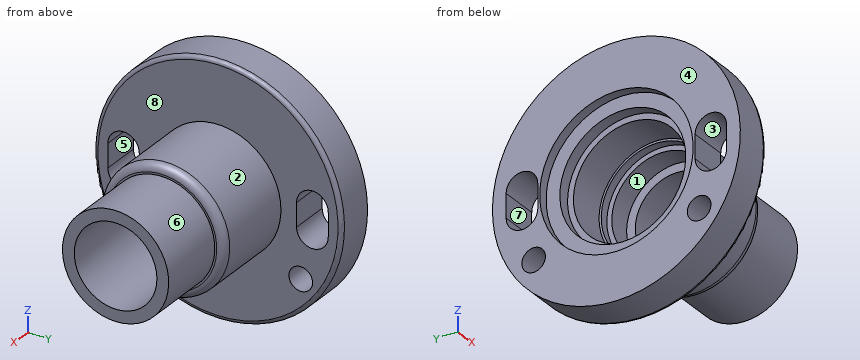
```python
from build123d import *

# Parameters (mm, degrees)
SKETCH1_R           = 31.5
BOSS_EXTRUDE1_DEPTH = 10
SKETCH2_R           = 16
BOSS_EXTRUDE2_DEPTH = 22
SKETCH3_R           = 13.5
BOSS_EXTRUDE3_DEPTH = 18
FILLET1_R           = 1
FILLET6_R           = 2
SKETCH4_R           = 10.5
CUT_EXTRUDE1_DEPTH  = 150
SKETCH5_R           = 12.7
CUT_EXTRUDE2_DEPTH  = 23.5
SKETCH6_R           = 13.95
CUT_EXTRUDE3_DEPTH  = 17.7
SKETCH7_R           = 14.5
CUT_EXTRUDE4_DEPTH  = 15.5
SKETCH8_R           = 16
CUT_EXTRUDE5_DEPTH  = 5.5
SKETCH9_R           = 19.5
CUT_EXTRUDE6_DEPTH  = 2.5
SKETCH10_R          = 3
CUT_EXTRUDE11_DEPTH = 20
SKETCH11_R          = 3
CUT_EXTRUDE12_DEPTH = 20
CUT_EXTRUDE16_DEPTH = 20
CUT_EXTRUDE17_DEPTH = 20


with BuildPart() as part:
    # Sketch1 → Boss-Extrude1 (new body)
    with BuildSketch(Plane(origin=(0, 0, 0), x_dir=(0, 0, -1), z_dir=(1, 0, 0))):
        Circle(SKETCH1_R)
    extrude(amount=BOSS_EXTRUDE1_DEPTH)

    # Sketch2 → Boss-Extrude2 (add)
    with BuildSketch(Plane(origin=(10, 0, 0), x_dir=(0, 0, -1), z_dir=(1, 0, 0))):
        Circle(SKETCH2_R)
    extrude(amount=BOSS_EXTRUDE2_DEPTH)

    # Sketch3 → Boss-Extrude3 (add)
    with BuildSketch(Plane(origin=(32, 0, 0), x_dir=(0, 0, -1), z_dir=(1, 0, 0))):
        Circle(SKETCH3_R)
    extrude(amount=BOSS_EXTRUDE3_DEPTH)

    # Fillet1
    fillet1_edges = [part.edges().sort_by_distance(p)[0] for p in [
        (10, 0, 31.5),
    ]]
    fillet(fillet1_edges, radius=FILLET1_R)

    # Fillet6
    fillet6_edges = [part.edges().sort_by_distance(p)[0] for p in [
        (32, 0, 16),
    ]]
    fillet(fillet6_edges, radius=FILLET6_R)

    # Sketch4 → Cut-Extrude1 (cut)
    with BuildSketch(Plane.ZY):
        Circle(SKETCH4_R)
    extrude(amount=-CUT_EXTRUDE1_DEPTH, mode=Mode.SUBTRACT)

    # Sketch5 → Cut-Extrude2 (cut)
    with BuildSketch(Plane.ZY):
        Circle(SKETCH5_R)
    extrude(amount=-CUT_EXTRUDE2_DEPTH, mode=Mode.SUBTRACT)

    # Sketch6 → Cut-Extrude3 (cut)
    with BuildSketch(Plane.ZY):
        Circle(SKETCH6_R)
    extrude(amount=-CUT_EXTRUDE3_DEPTH, mode=Mode.SUBTRACT)

    # Sketch7 → Cut-Extrude4 (cut)
    with BuildSketch(Plane.ZY):
        Circle(SKETCH7_R)
    extrude(amount=-CUT_EXTRUDE4_DEPTH, mode=Mode.SUBTRACT)

    # Sketch8 → Cut-Extrude5 (cut)
    with BuildSketch(Plane.ZY):
        with Locations(Location((0, 0, 0), (0, 0, 180))):
            Circle(SKETCH8_R)
    extrude(amount=-CUT_EXTRUDE5_DEPTH, mode=Mode.SUBTRACT)

    # Sketch9 → Cut-Extrude6 (cut)
    with BuildSketch(Plane.ZY):
        Circle(SKETCH9_R)
    extrude(amount=-CUT_EXTRUDE6_DEPTH, mode=Mode.SUBTRACT)

    # Sketch10 → Cut-Extrude11 (cut)
    with BuildSketch(Plane(origin=(10, 0, 0), x_dir=(0, 0, -1), z_dir=(1, 0, 0))):
        with Locations((15.279966328, 21.0310694)):
            Circle(SKETCH10_R)
    extrude(amount=-CUT_EXTRUDE11_DEPTH, mode=Mode.SUBTRACT)

    # Sketch11 → Cut-Extrude12 (cut)
    with BuildSketch(Plane.ZY):
        with Locations((-15.28241656, -21.034441854)):
            Circle(SKETCH11_R)
    extrude(amount=-CUT_EXTRUDE12_DEPTH, mode=Mode.SUBTRACT)

    # Sketch12 → Cut-Extrude16 (cut)
    with BuildSketch(Plane.ZY):
        with BuildLine():
            Line((-3, -20.009180996), (3, -20.009180996))
            ThreePointArc((3, -20.009180996), (6.990819004, -24), (3, -27.990819004))
            Line((3, -27.990819004), (-3, -27.990819004))
            ThreePointArc((-3, -27.990819004), (-6.990819004, -24), (-3, -20.009180996))
        make_face()
    extrude(amount=-CUT_EXTRUDE16_DEPTH, mode=Mode.SUBTRACT)

    # Sketch14 → Cut-Extrude17 (cut)
    with BuildSketch(Plane.ZY):
        with BuildLine():
            Line((-3, 28.020849302), (3, 28.020849302))
            ThreePointArc((3, 28.020849302), (7.020849302, 24), (3, 19.979150698))
            Line((3, 19.979150698), (-3, 19.979150698))
            ThreePointArc((-3, 19.979150698), (-7.020849302, 24), (-3, 28.020849302))
        make_face()
    extrude(amount=-CUT_EXTRUDE17_DEPTH, mode=Mode.SUBTRACT)


solid = part.part
```
CAD build for the part. Positions are in the model's coordinates, mm. Face numbers are marked on the shaded views. A direction names the side the tool comes from. Round coordinates to 2 decimals unless told otherwise and drop trailing zeros. Write each loop counter-clockwise with the first axis right and the second up, starting at its lowest first coordinate (ties: lowest second). Pieces come first, ordered by that corner, then holes. Notation, with made-up numbers: (-33, 25.25) -> (22, 25.25) arc R7 cw to (22, 32.25) -> close; hole circle Ø11 at (76, 75.5). An arc over 180 degrees is marked (long way). Answer in a Markdown table with one row per item. Add a question column.
Item 1: Saw through at A-A, the plane x = 36. Write the cut outline in (y, z).
Item 2: Drop flat-ended pins along their axis: pin 1 Ø3 at (x, z) = (4.5, -1) entering from +Y; pin 2 Ø6 at (y, z) = (-10.5, 13) entering from +X; pin 3 Ø1 at (y, z) = (6.5, -14) entering from -X; pin 4 Ø20.5 at (y, z) = (0, 0) entering from +X. Give the stop position or say it passes through.
Item 3: Drill centre lines: line 1 (Y direction, x = 4, z = 0); line 2 (Y direction, x = 1.8, z = 0); line 3 (Y direction, x = 20, z = 0). Where is each one in solid material? Low to high. Write a range as from..to.
Item 4: Which spindle directions (+Z, -Z, +X, -X, +Y, -Y) get a long thin tool onto all of the face, cutting with end or side? Do the marked faces 1, 2, 3 and 4. Say none if no direction does.
Item 5: Saw through at B-B, the plane z = 0. Count the separate pieces of the cut face and the enclosed holes in it, then the cut area to 3 significant figures.
Item 6: Mould opens along Z. For the marked faces 5, 6, 7 and 8 say: pulls with the +Z half, pulls with the -Z half, needs draft (parallel to the pull), parting line crosses it, or undercut.
Item 7: Saw through at C-C, the plane x = 20. Write the cut outline in (y, z).
Findings below:
| question | item | result |
|---|---|---|
| 1 | outline | circle Ø27 at (0, 0); hole circle Ø21 at (0, 0) |
| 2 | pin 1 | stops at y = 31.5 |
| 2 | pin 2 | stops at x = 32 |
| 2 | pin 3 | stops at x = 5.5 |
| 2 | pin 4 | passes through |
| 3 | line 1 | y = -31.5..-27.99, -20.01..-16, 16..19.98, 28.02..31.5 |
| 3 | line 2 | y = -31.5..-27.99, -20.01..-19.5, 19.5..19.98, 28.02..31.5 |
| 3 | line 3 | y = -16..-12.7, 12.7..16 |
| 4 | face 1 | -X |
| 4 | face 2 | +X |
| 4 | face 3 | +X, -X |
| 4 | face 4 | +Z, -Z, -X, +Y, -Y |
| 5 | separate pieces | 4 |
| 5 | enclosed holes | 0 |
| 5 | area | 409 mm^2 |
| 6 | face 5 | undercut |
| 6 | face 6 | parting line crosses it |
| 6 | face 7 | undercut |
| 6 | face 8 | needs draft |
| 7 | outline | circle Ø32 at (0, 0); hole circle Ø25.4 at (0, 0) |
